For this review, take the finished solid that the model builds, in its own axes (mm). Round coordinates to 2 decimals unless told otherwise and drop trailing zeros. Order: outer loops, then holes, each group sorted by start corner. A loop starts at its lowest first (then second) coordinate and runs counter-clockwise, first axis right, second up. Notation, with made-up numbers: M 25,9.25 L 38,9.25 A19 cw 38,17.25 Z; hole C 46,60 d3. An arc over 180 degrees is marked long. Use a Markdown table: item, result.
from build123d import *

# Parameters (mm, degrees)
SKETCH1_R           = 2.5
BOSS_EXTRUDE1_DEPTH = 2
CHAMFER1_SIZE       = 0.2


with BuildPart() as part:
    # Sketch1 → Boss-Extrude1 (new body)
    with BuildSketch(Plane.XY):
        Polygon((0, 4.734272207), (-4.1, 2.367136104), (-4.1, -2.367136104), (0, -4.734272207), (4.1, -2.367136104), (4.1, 2.367136104), align=None)
        Circle(SKETCH1_R, mode=Mode.SUBTRACT)
    extrude(amount=BOSS_EXTRUDE1_DEPTH)

    # Chamfer1
    chamfer1_edges = [part.edges().sort_by_distance(p)[0] for p in [
        (-2.5, 0, 0),
        (-2.5, 0, 2),
    ]]
    chamfer(chamfer1_edges, length=CHAMFER1_SIZE)


solid = part.part
Q1. Add section A-A (y = 0). Write out the cut boundary in (x, z), then the cut area to 3 significant figures.
Determined:
| item | result |
|---|---|
| outline | M -4.1,0 L -2.7,0 L -2.5,0.2 L -2.5,1.8 L -2.7,2 L -4.1,2 Z; M 2.5,0.2 L 2.7,0 L 4.1,0 L 4.1,2 L 2.7,2 L 2.5,1.8 Z |
| area | 6.32 mm^2 |
Q2. Draft analysis for pull direction Y (two halves, no side actions). For faces 1 (the cylindrical face through (-0.54, -2.44, 0.99)), 2 (the flat face through (2.079, 3.534, 0.986)), 3 (the flat face through (-3, 0, 0)), 4 (the flat face through (2.02, -3.57, 0.99)), state which applies: pulls with the +Y half, pulls with the -Y half, needs draft (parallel to the pull), parting line crosses it, or undercut.
Determined:
| item | result |
|---|---|
| face 1 | undercut |
| face 2 | pulls with the +Y half |
| face 3 | needs draft |
| face 4 | pulls with the -Y half |
Q3. Wall thickness on line 1 along Y through (x, z) = (2, 0.55); line 2 along Y through (x, z) = (-2.25, 1); line 3 along X through (y, z) = (1, 0.15): over which ranges is each line inside the solid? List them lowest first. Write a range as [from, to].
Determined:
| item | result |
|---|---|
| line 1 | y = [-3.58, -1.5], [1.5, 3.58] |
| line 2 | y = [-3.44, -1.09], [1.09, 3.44] |
| line 3 | x = [-4.1, -2.35], [2.35, 4.1] |
Q4. Add section B-B (z = 0.6). Write out the cut boundary in (x, y).
Determined:
| item | result |
|---|---|
| outline | M -4.1,-2.37 L 0,-4.73 L 4.1,-2.37 L 4.1,2.37 L 0,4.73 L -4.1,2.37 Z; hole C 0,0 d5 |
Q5. Clearance check with a flat-ended pin moving along its axis: pin 1 (1.5 mm diameter, centred on x = -0.5, y = -2, fed in from +Z). State where the tip first meets the part, or that it passes through.
Determined:
| item | result |
|---|---|
| pin 1 | stops at z = 2 |
Q6. Add section D-D (x = -3.25). Write out the cut boundary in (y, z).
Determined:
| item | result |
|---|---|
| outline | M -2.86,0 L 2.86,0 L 2.86,2 L -2.86,2 Z |
Q7. Add section C-C (y = 4). Write out the cut boundary in (x, z), then the cut area to 3 significant figures.
Determined:
| item | result |
|---|---|
| outline | M -1.27,0 L 1.27,0 L 1.27,2 L -1.27,2 Z |
| area | 5.09 mm^2 |
